The listing builds one solid part. Answer for the finished solid, in the listing's coordinates (mm). Face numbers are marked on the shaded views. A direction names the side the tool comes from. Coordinates: 2 decimals unless noted, no trailing zeros. Order: outer loops, then holes, each group sorted by start corner. A loop starts at its lowest first (then second) coordinate and runs counter-clockwise, first axis right, second up. Notation, with made-up numbers: (59.25, 36) -> (91.25, 36) arc R19 cw to (91.25, 51) -> close; hole circle Ø6 at (-19.5, 19.25). An arc over 180 degrees is marked (long way). Return JSON: item names as keys, results as strings.
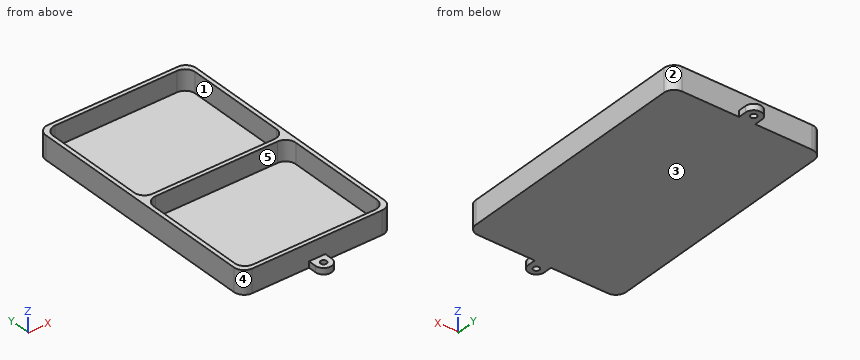
Autodesk Inventor part; units mm, degrees
ref_plane "YZ Plane" through (0, 0, 0) normal (1, 0, 0) x (0, 1, 0)
ref_plane "XZ Plane" through (0, 0, 0) normal (0, 1, 0) x (-1, 0, 0)
ref_plane "XY Plane" through (0, 0, 0) normal (0, 0, 1) x (1, 0, 0)
sketch "Sketch1" plane through (0, 0, 0) normal (0, 0, 1) x (1, 0, 0)
  line L0 (-37, -63) -> (37, -63)
  line L1 (37, -63) -> (37, 63)
  line L2 (37, 63) -> (-37, 63)
  line L3 (-37, 63) -> (-37, -63)
  line L4 (-37, -63) -> (37, 63) construction
  line L5 (37, -63) -> (-37, 63) construction
  point P0 (0, 0)
  dimension "d0" = 74
  dimension "d1" = 126
extrude "Extrusion1" add sketch "Sketch1" along normal blind 1.5
sketch "Sketch2" plane through (0, 0, 1.5) normal (0, 0, 1) x (1, 0, 0)
  line L0 (37, -63) -> (37, 63)
  line L1 (-37, -63) -> (37, -63)
  line L2 (37, -63) -> (37, 63)
  line L3 (37, 63) -> (-37, 63)
  line L4 (-37, 63) -> (-37, -63)
  line L5 (-37, -63) -> (37, 63) construction
  line L6 (37, -63) -> (-37, 63) construction
  line L7 (-35, -61) -> (35, -61)
  line L8 (35, -61) -> (35, 61)
  line L9 (35, 61) -> (-35, 61)
  line L10 (-35, 61) -> (-35, -61)
  line L11 (-35, -61) -> (35, 61) construction
  line L12 (35, -61) -> (-35, 61) construction
  line L13 (-35, -1) -> (35, -1)
  line L14 (35, -1) -> (35, 1)
  line L15 (35, 1) -> (-35, 1)
  line L16 (-35, 1) -> (-35, -1)
  line L17 (-35, -1) -> (35, 1) construction
  line L18 (35, -1) -> (-35, 1) construction
  point P0 (0, 0)
  dimension "d4" = 70
  dimension "d5" = 122
  dimension "d6" = 2
extrude "Extrusion2" add sketch "Sketch2" along normal blind 10 contours L1 L4 L3 L0 | L10 L15 L8 L13
fillet "Fillet1" radius 5 12 edges at (37, 63, 5.75) (-37, 63, 5.75) (37, -63, 5.75) (-37, -63, 5.75) (-35, 61, 6.5) (35, 61, 6.5) (35, 1, 6.5) (35, -1, 6.5) (-35, 1, 6.5) (-35, -1, 6.5) (-35, -61, 6.5) (35, -61, 6.5)
sketch "Sketch3" plane through (0, 0, 0) normal (0, 0, -1) x (-1, 0, 0)
  line L0 (-32, 63) -> (32, 63)
  line L1 (0, 63) -> (0, 71)
  circle A0 centre (0, 67) radius 4
  circle A1 centre (0, 67) radius 1.5
  line L2 (-4, 67) -> (4, 67)
  line L3 (4, 67) -> (4, 63)
  line L4 (-4, 67) -> (-4, 63)
  line L5 (-53.0047, 0) -> (53.0047, 0)
  line L6 (-30, 1) -> (30, 1)
  line L7 (0, -63) -> (0, -71)
  circle A2 centre (0, -67) radius 4
  circle A3 centre (0, -67) radius 1.5
  line L8 (-4, -67) -> (4, -67)
  line L9 (4, -67) -> (4, -63)
  line L10 (-4, -67) -> (-4, -63)
  line L11 (-30, -1) -> (30, -1)
  line L12 (4, -63) -> (-4, -63)
  line L13 (32, -63) -> (-32, -63)
  point P0 (0, 0)
  dimension "d11" = 8
  dimension "d10" = 8
  dimension "d12" = 3
extrude "Extrusion3" add sketch "Sketch3" against normal blind 3 contours L4 A0 L0 | A0 L3 L0 | A0 L2 A1 L1 | L1 A1 L2 A0 | A0 L1 A1 L2 | L2 A1 L1 A0 | A2 L8 A3 L7 | L12 L9 A2 | L7 A3 L8 A2 | A2 L10 L12 | A2 L7 A3 L8 | L8 A3 L7 A2
properties part number "box store"
1. The part is cut by section C-C on x = -13. Give the vertices of the cut face in (y, z).
Answer block:
{"outline": "(-63, 0) -> (63, 0) -> (63, 11.5) -> (61, 11.5) -> (61, 1.5) -> (1, 1.5) -> (1, 11.5) -> (-1, 11.5) -> (-1, 1.5) -> (-61, 1.5) -> (-61, 11.5) -> (-63, 11.5) -> close"}
2. The part is cut by section A-A on y = 37. Give the vertices of the cut face in (x, z).
Answer block:
{"outline": "(-37, 0) -> (37, 0) -> (37, 11.5) -> (35, 11.5) -> (35, 1.5) -> (-35, 1.5) -> (-35, 11.5) -> (-37, 11.5) -> close"}
3. Each of these flat-tipped pins is pushed along its axis until it touches: pin 1 Ø4 at (x, y) = (0.5, -65.5) entering from +Z; pin 2 Ø1.5 at (y, z) = (66, 1) entering from -X; pin 3 Ø2.5 at (y, z) = (-64.5, 1.5) entering from +X. Where does it stop, or does it pass through?
Answer block:
{"pin 1": "stops at z = 3", "pin 2": "stops at x = -4", "pin 3": "stops at x = 4"}
4. Consider line 1 (Y direction, x = 0, z = 1.65); line 2 (Y direction, x = 19, z = 8); line 3 (Y direction, x = 0, z = 0.7). Determine where each line is inside the solid, lowest interval first. Write a range as from..to.
Answer block:
{"line 1": "y = -71..-68.5, -65.5..-61, -1..1, 61..65.5, 68.5..71", "line 2": "y = -63..-61, -1..1, 61..63", "line 3": "y = -71..-68.5, -65.5..65.5, 68.5..71"}
5. For the marked faces 1 and 2, determine the directions among +Z, -Z, +X, -X, +Y, -Y from which every point of the face is accessible in a straight line to the end or side of a thin tool.
Answer block:
{"face 1": "+Z", "face 2": "+Z, -Z, +X, +Y"}
6. The part is cut by section B-B on z = 6. Give the vertices of the cut face in (x, y), and give its area (3 significant figures).
Answer block:
{"outline": "(-37, -58) arc R5 ccw to (-32, -63) -> (32, -63) arc R5 ccw to (37, -58) -> (37, 58) arc R5 ccw to (32, 63) -> (-32, 63) arc R5 ccw to (-37, 58) -> close; hole (-35, -56) arc R5 ccw to (-30, -61) -> (30, -61) arc R5 ccw to (35, -56) -> (35, -6) arc R5 ccw to (30, -1) -> (-30, -1) arc R5 ccw to (-35, -6) -> close; hole (-35, 6) arc R5 ccw to (-30, 1) -> (30, 1) arc R5 ccw to (35, 6) -> (35, 56) arc R5 ccw to (30, 61) -> (-30, 61) arc R5 ccw to (-35, 56) -> close", "area": "945 mm2"}
7. Determine the mould class of the marked faces 3, 4 and 5 for opening direction Y: pulls with the +Y half, pulls with the -Y half, needs draft (parallel to the pull), parting line crosses it, or undercut.
Answer block:
{"face 3": "needs draft", "face 4": "pulls with the -Y half", "face 5": "undercut"}
